```python
from build123d import *

# Parameters (mm, degrees)
F1_DEPTH = 47.625
F2_R     = 15.875
F3_DEPTH = 15.875
F4_R     = 6.35
F5_DEPTH = 34.29


with BuildPart() as f1:
    # F0 (on Front) → F1 (new body)
    with BuildSketch(Plane.XZ):
        with BuildLine():
            ThreePointArc((-52.3875, 31.75), (-84.1375, 0), (-52.3875, -31.75))
            Line((-52.3875, -31.75), (52.3875, -31.75))
            Line((52.3875, -31.75), (52.3875, 0))
            ThreePointArc((52.3875, 0), (29.93686, 9.29936), (20.6375, 31.75))
            Line((20.6375, 31.75), (-52.3875, 31.75))
        make_face()
    extrude(amount=F1_DEPTH)

    # F2 (on face) → F3 (cut)
    with BuildSketch(Plane.XZ.offset(47.625)):
        with Locations((-52.3875, 0)):
            Circle(F2_R)
    extrude(amount=-F3_DEPTH, mode=Mode.SUBTRACT)

    # F4 (on face) → F5 (cut)
    with BuildSketch(Plane.XZ.offset(31.75)):
        with Locations((-52.3875, 0)):
            Circle(F4_R)
    extrude(amount=-F5_DEPTH, mode=Mode.SUBTRACT)


solid = f1.part
```
Model file for the job. Use its own axes, mm. A direction names the side the tool comes from. Give positions to 0.01 mm unless a question says otherwise; leave off trailing zeros. Write each loop counter-clockwise with the first axis right and the second up, starting at its lowest first coordinate (ties: lowest second). Pieces come first, ordered by that corner, then holes. Notation, with made-up numbers: (26, -17) - (71, -17) arc R26 cw to (71, 20) - close; hole circle Ø1 at (-18.75, 27.25). An arc over 180 degrees is marked (long way). One line per question, with ' | ' between items. Start each with the question number.
(1) Slice it at A-A on z = 5. Write the cut outline in (x, y) (3 decimals), plus the area to 3 significant figures.
(2) Slice it at C-C on x = -66.5. Write the cut outline in (y, z) (3 decimals).
(3) Wall check: line 1 along X through (y, z) = (-7.5, -0.5); line 2 along Y through (x, z) = (-48, 13.5); line 3 along Z through (x, y) = (-47.5, -14.5). Give the ranges that are in metal, low to high. Write a range as from..to.
(4) 3-axis set-ups, long thin cutter, end or side, ignore diameter. For faces 1 (the face through (-55.829, -39.799, -15.497)), 2 (the face through (-46.33, -16.1, 1.91)): which of +Z, -Z, +X, -X, +Y, -Y reach the whole face in a straight line?
(5) Pin check, flat tips, straight feed: P1, Ø12, axis at x = -70.5, y = -13, coming from the -Z side; P2, Ø1.5, axis at x = -62.5, y = -5, coming from the -Z side; P3, Ø14.5, axis at x = -52.39, z = 0, coming from the -Y side. Stop position of each tip, or through.
(6) Slice it at B-B on y = -7. Write the cut outline in (x, z), plus the area to 3 significant figures.
(7) Two-plate mould, pull along X, no slides. Class faces 3 (the face through (-45.6, -31.75, 0.2)), 4 (the face through (-1, -23, -31.75)), 5 (the face through (52.388, -23, -16)): +X half, -X half, draft (parallel to the pull), parting line (faces both ways), or undercut.
Results below:
1) outline: (-83.741, -47.625) - (-67.455, -47.625) - (-67.455, -31.75) - (-56.302, -31.75) - (-56.302, 0) - (-83.741, 0) - close; (-48.473, -31.75) - (-37.32, -31.75) - (-37.32, -47.625) - (35.285, -47.625) - (35.285, 0) - (-48.473, 0) - close | area: 4,940 mm^2
2) outline: (-47.625, -28.441) - (0, -28.441) - (0, 28.441) - (-47.625, 28.441) - (-47.625, 7.27) - (-31.75, 7.27) - (-31.75, -7.27) - (-47.625, -7.27) - close
3) line 1: -84.13..-58.72, -46.06..52.39 | line 2: -31.75..0 | line 3: -31.75..-4.05, 4.05..31.75
4) face 1: -Y | face 2: +Y, -Y
5) P1: z = -29.35 | P2: z = -30.34 | P3: y = -31.75
6) outline: (-52.39, -31.75) - (52.39, -31.75) - (52.39, 0) arc R31.75 cw to (20.64, 31.75) - (-52.39, 31.75) arc R31.75 ccw to start; hole circle Ø12.7 at (-52.39, 0) | area: 7,320 mm^2
7) face 3: undercut | face 4: draft | face 5: +X half
